Could you check a few things on this model? Use its own coordinates, in mm. Face numbers are marked on the shaded views. A direction names the side the tool comes from. Give positions to 0.01 mm unless a question says otherwise; leave off trailing zeros. Loops run counter-clockwise (first coordinate to the right, second up) from the corner with the lowest first, then second, coordinate; pieces in that order, holes last.
1. I need wall thicknesses on line 1 along X through (y, z) = (5.25, 23); line 2 along Z through (x, y) = (-3, 8); line 3 along Z through (x, y) = (6.5, 2.5). Which ranges of each line are inside material? Lowest first, please.
2. Imagine slicing it at B-B (z = 40). List the corners of the cut face in (x, y) for me, plus the area to 3 significant figures.
3. Imagine slicing it at D-D (x = 22). List the corners of the cut face in (y, z) for me.
4. Imagine slicing it at A-A (y = 4.5). List the corners of the cut face in (x, z) for me, plus the area to 3 significant figures.
5. For P1, Ø14, axis at x = -0.5, z = 25, coming from the -Y side; P2, Ø8, axis at x = -20, z = 13, coming from the +Y side, each with a flat end and sliding along its axis, tell me the tip position at first contact or that it passes through.
6. Thinking about a two-plate mould opening in X: for the marked faces 1, 2 and 3, which applies, +X half, -X half, draft (parallel to the pull), parting line (faces both ways), or undercut?
7. For the marked faces 4 and 5, which set-ups out of +Z, -Z, +X, -X, +Y, -Y let a thin tool reach every point of the face, with its end or its side?
8. Imagine slicing it at C-C (z = 6). List the corners of the cut face in (x, y) for me.
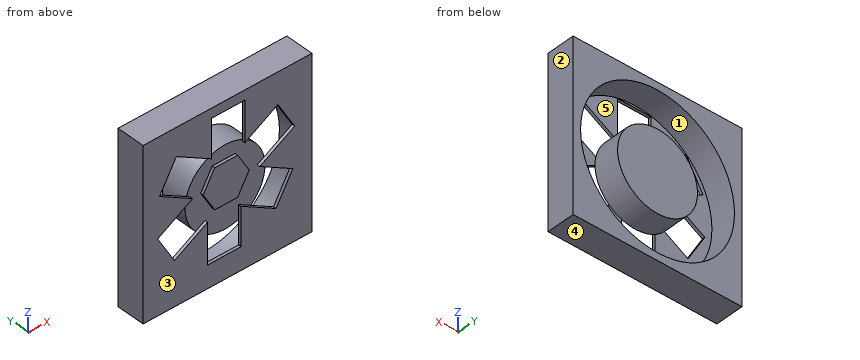
```python
from build123d import *

# Parameters (mm, degrees)
SKETCH1_W           = 60
SKETCH1_H           = 60
BOSS_EXTRUDE1_DEPTH = 10
SKETCH2_R           = 27.339129043
SKETCH2_R_2         = 14.209467058
CUT_EXTRUDE1_DEPTH  = 9
SKETCH3_W           = 11.919517594
SKETCH3_H           = 17.209998666
SKETCH3_W_2         = 11.919517595
CUT_EXTRUDE3_DEPTH  = 1


with BuildPart() as part:
    # Sketch1 → Boss-Extrude1 (new body)
    with BuildSketch(Plane(origin=(0, 0, 0), x_dir=(1, 0, 0), z_dir=(0, 1, 0))):
        with Locations((-3.583333333, -23)):
            Rectangle(SKETCH1_W, SKETCH1_H)
    extrude(amount=BOSS_EXTRUDE1_DEPTH)

    # Sketch2 → Cut-Extrude1 (cut)
    with BuildSketch(Plane(origin=(0, 10, 0), x_dir=(1, 0, 0), z_dir=(0, 1, 0))):
        with Locations((-3.583333333, -23)):
            Circle(SKETCH2_R)
        with Locations((-3.583333333, -23)):
            Circle(SKETCH2_R_2, mode=Mode.SUBTRACT)
    extrude(amount=-CUT_EXTRUDE1_DEPTH, mode=Mode.SUBTRACT)

    # Sketch3 → Cut-Extrude3 (cut)
    with BuildSketch(Plane.XZ):
        Polygon((14.324988363, 42.018967665), (-0.579307681, 33.413968332), (5.380451117, 23.091363294), (20.284747161, 31.696362627), align=None)
        with Locations((-3.392111126, 40.974887496)):
            Rectangle(SKETCH3_W, SKETCH3_H)
        Polygon((19.615469435, 17.733747325), (4.711173391, 26.338746658), (-1.248585407, 16.01614162), (13.655710637, 7.411142287), align=None)
        with Locations((-4.730666578, 9.614445482)):
            Rectangle(SKETCH3_W_2, SKETCH3_H)
        Polygon((-22.447766067, 8.570365313), (-7.543470023, 17.175364646), (-13.50322882, 27.497969684), (-28.407524864, 18.892970351), align=None)
        Polygon((-27.738247138, 32.855585653), (-12.833951095, 24.25058632), (-6.874192297, 34.573191357), (-21.778488341, 43.178190691), align=None)
    extrude(amount=-CUT_EXTRUDE3_DEPTH, mode=Mode.SUBTRACT)


solid = part.part
```
Derived:
1. line 1: x = -33.58 to -30.92, -17.79 to 10.63, 23.76 to 26.42
1. line 2: z = -7 to -4.33, 8.8 to 37.2, 50.33 to 53
1. line 3: z = -7 to -2.41, 12.99 to 33.01, 48.41 to 53
2. outline: (-33.58, 0) - (-23.61, 0) - (-23.61, 1) - (-24.99, 1) - (-24.99, 10) - (-33.58, 10) - close; (-16.27, 0) - (-9.35, 0) - (-9.35, 1) - (-16.27, 1) - close; (2.57, 0) - (10.83, 0) - (10.83, 1) - (2.57, 1) - close; (15.49, 0) - (26.42, 0) - (26.42, 10) - (17.83, 10) - (17.83, 1) - (15.49, 1) - close
2. area: 191 mm2
3. outline: (0, -7) - (10, -7) - (10, 13.36) - (1, 13.36) - (1, 32.64) - (10, 32.64) - (10, 53) - (0, 53) - close
4. outline: (-33.58, -7) - (26.42, -7) - (26.42, 53) - (-33.58, 53) - close; circle Ø28.42 at (-3.58, 23); hole circle Ø54.68 at (-3.58, 23)
4. area: 1,890 mm2
5. P1: stops at y = 0
5. P2: stops at y = 1
6. face 1: undercut
6. face 2: +X half
6. face 3: draft
7. face 4: -Z, +X, -X, +Y, -Y
7. face 5: +Y
8. outline: (-33.58, 0) - (-10.69, 0) - (-10.69, 1) - (-24.99, 1) - (-24.99, 10) - (-33.58, 10) - close; (1.23, 0) - (26.42, 0) - (26.42, 10) - (17.83, 10) - (17.83, 1) - (1.23, 1) - close
